```python
from build123d import *


with BuildPart() as part:
    # Sketch1 → Revolve1 (revolve)
    with BuildSketch(Plane.XY, mode=Mode.PRIVATE) as revolve1_sk:
        with BuildLine():
            Line((6640.084580843, 3596.961198709), (6640.084580843, 3502.981198709))
            ThreePointArc((6640.084580843, 3502.981198709), (6610.286564464, 3523.770326487), (6619.510580843, 3558.913279348))
            Line((6619.510580843, 3558.913279348), (6619.510580843, 3562.400142715))
            Line((6619.510580843, 3562.400142715), (6622.685580843, 3562.400142715))
            Line((6622.685580843, 3562.400142715), (6622.685580843, 3568.750142715))
            Line((6622.685580843, 3568.750142715), (6619.510580843, 3568.750142715))
            Line((6619.510580843, 3568.750142715), (6619.510580843, 3585.338770448))
            Line((6619.510580843, 3585.338770448), (6622.685580843, 3585.338770448))
            Line((6622.685580843, 3585.338770448), (6622.685580843, 3591.688770448))
            Line((6622.685580843, 3591.688770448), (6619.510580843, 3591.688770448))
            Line((6619.510580843, 3591.688770448), (6619.510580843, 3596.961198709))
            Line((6619.510580843, 3596.961198709), (6640.084580843, 3596.961198709))
        make_face()
    revolve(revolve1_sk.sketch.rotate(Axis((6640.084580843, 3596.961198709, 0), (0, -1, 0)), 270), axis=Axis((6640.084580843, 3596.961198709, 0), (0, -1, 0)))


solid = part.part
```
Check sheet for the modelled part. Datum: model origin and axes. Units: mm. A direction names the side the tool comes from. Give positions to 0.01 mm unless a question says otherwise; leave off trailing zeros. Order: outer loops, then holes, each group sorted by start corner. A loop starts at its lowest first (then second) coordinate and runs counter-clockwise, first axis right, second up. Notation, with made-up numbers: (44.25, -29) -> (97.25, -29) arc R18 ccw to (97.25, 3) -> close; hole circle Ø5 at (37.25, 45). An arc over 180 degrees is marked (long way). Return JSON: item names as keys, results as strings.
1. Cross-section at D-D, the plane z = -24. Record the cut outline in (x, y), plus the area to 3 significant figures.
From the geometry:
{"outline": "circle Ø41.57 at (6640.08, 3534.73)", "area": "1,360 mm^2"}
2. Cross-section at C-C, the plane y = 3526. Record the cut outline in (x, z), plus the area to 3 significant figures.
From the geometry:
{"outline": "circle Ø61.05 at (6640.08, 0)", "area": "2,930 mm^2"}
3. Set-up check for faces 4 (the flat face through (6635, 3562.4, -17)), 5 (the cylindrical face through (6660.17, 3594.36, -4.46)): record each of +Z, -Z, +X, -X, +Y, -Y from which the full face is reachable in a straight line by a thin tool's end or side.
From the geometry:
{"face 4": "none", "face 5": "+Y"}
4. Cross-section at B-B, the plane x = 6649. Record the cut outline in (y, z).
From the geometry:
{"outline": "(3558.91, -18.54) -> (3562.4, -18.54) -> (3562.4, -14.94) -> (3568.75, -14.94) -> (3568.75, -18.54) -> (3585.34, -18.54) -> (3585.34, -14.94) -> (3591.69, -14.94) -> (3591.69, -18.54) -> (3596.96, -18.54) -> (3596.96, 18.54) -> (3591.69, 18.54) -> (3591.69, 14.94) -> (3585.34, 14.94) -> (3585.34, 18.54) -> (3568.75, 18.54) -> (3568.75, 14.94) -> (3562.4, 14.94) -> (3562.4, 18.54) -> (3558.91, 18.54) arc R30.47 ccw (long way) to start"}
5. Cross-section at A-A, the plane z = 0. Record the cut outline in (x, y).
From the geometry:
{"outline": "(6619.51, 3558.91) arc R31.75 ccw (long way) to (6660.66, 3558.91) -> (6660.66, 3562.4) -> (6657.48, 3562.4) -> (6657.48, 3568.75) -> (6660.66, 3568.75) -> (6660.66, 3585.34) -> (6657.48, 3585.34) -> (6657.48, 3591.69) -> (6660.66, 3591.69) -> (6660.66, 3596.96) -> (6619.51, 3596.96) -> (6619.51, 3591.69) -> (6622.69, 3591.69) -> (6622.69, 3585.34) -> (6619.51, 3585.34) -> (6619.51, 3568.75) -> (6622.69, 3568.75) -> (6622.69, 3562.4) -> (6619.51, 3562.4) -> close"}
6. Mould release check, pull along Y, two halves, no side actions. Record for faces 1 (the flat face through (6640, 3596.961, 0)), 2 (the flat face through (6635, 3591.689, 17)), 3 (the cylindrical face through (6660.17, 3560.68, -4.46)): +Y half, -Y half, draft (parallel to the pull), parting line (faces both ways), or undercut.
From the geometry:
{"face 1": "+Y half", "face 2": "undercut", "face 3": "draft"}
7. Go/stop test with flat-tipped pins: P1, Ø4, axis at x = 6634, y = 3534.5, coming from the -Z side; P2, Ø2, axis at x = 6651, y = 3539.5, coming from the +Z side; P3, Ø4, axis at x = 6644.5, z = 13.5, coming from the -Y side. Record where each tip stops, or that it passes through.
From the geometry:
{"P1": "z = -31.49", "P2": "z = 29.82", "P3": "y = 3505.42"}
8. Material ranges on probe 1 along Y at (x, z) = (6624.5, 12); probe 2 along X at (y, z) = (3580.5, 11); probe 3 along Z at (x, y) = (6638, 3582.5), recorded low to high. Write a range as [from, to].
From the geometry:
{"probe 1": "[3509.81, 3562.4], [3568.75, 3585.34], [3591.69, 3596.96]", "probe 2": "[6622.7, 6657.47]", "probe 3": "[-20.47, 20.47]"}
